Design review of the part built by this model. Coordinates are the model's own, in mm. Face numbers are marked on the shaded views. Give positions to 0.01 mm unless a question says otherwise; leave off trailing zeros. Loops run counter-clockwise (first coordinate to the right, second up) from the corner with the lowest first, then second, coordinate; pieces in that order, holes last. Notation, with made-up numbers: (-20, 88) -> (38, 88) arc R12 ccw to (38, 98) -> close; hole circle Ø11 at (18, 11). An arc over 180 degrees is marked (long way). Answer in a Markdown table with one row per item. Add a question column.
(1) Consider section D-D on x = -83. Write out the cut boundary in (y, z), then the cut area to 3 significant figures.
(2) Draft analysis for pull direction Y (two halves, no side actions). For the marked faces 1, 2 and 3, state which applies: +Y half, -Y half, draft (parallel to the pull), parting line (faces both ways), or undercut.
(3) Consider section B-B on x = -36.5. Write out the cut boundary in (y, z), then the cut area to 3 significant figures.
(4) Consider section A-A on y = -30. Write out the cut boundary in (x, z).
(5) For pin 1 (4 mm diameter, centred on x = 70.5, y = 35, fed in from -Z); pin 2 (4 mm diameter, centred on x = -32.5, y = 17.5, fed in from -Z); pin 3 (2 mm diameter, centred on y = -23.5, z = -3, fed in from +X), all flat-tipped, find the tip position at first contact; note any pin that passes through.
(6) For line 1 (Y direction, x = 32.5, z = 8.5); line 2 (Z direction, x = -15, y = 40.5); line 3 (X direction, y = 10.5, z = 6), list the stretches that pass through material, from the lowest coordinate up.
(7) Consider section C-C on y = 17. Write out the cut boundary in (x, z).
from build123d import *

# Parameters (mm, degrees)
BOSS_EXTRUDE1_DEPTH    = 13
SKETCH3_R              = 1.65
SKETCH3_R_2            = 1.5
CUT_EXTRUDE1_DEPTH     = 14
SKETCH4_W              = 13
SKETCH4_H              = 83
BOSS_EXTRUDE2_DEPTH    = 5
BOSS_EXTRUDE3_DEPTH    = 1
FILLET1_R              = 2
HOLE_WIZARD_M3_1_D     = 2.5
HOLE_WIZARD_M3_1_DEPTH = 12
HOLE_WIZARD_M3_1_TIP   = 0.751075774
CUT_EXTRUDE_1_DEPTH    = 17


with BuildPart() as part:
    # Sketch1 → Boss-Extrude1 (new body)
    with BuildSketch(Plane.XY):
        Polygon((-95, 44), (-35, 44), (95, 44), (95, -44), (-95, -44), align=None)
    extrude(amount=BOSS_EXTRUDE1_DEPTH)

    # Sketch3 → Cut-Extrude1 (cut, through all)
    with BuildSketch(Plane.XY.offset(13)):
        with Locations((-58.6, -41.5)):
            Circle(SKETCH3_R)
        with Locations((-23.6, -41.5)):
            Circle(SKETCH3_R)
        with Locations((11.4, -41.5)):
            Circle(SKETCH3_R)
        with Locations((32.5, -41.5)):
            Circle(SKETCH3_R_2)
        with Locations((77.5, -41.5)):
            Circle(SKETCH3_R_2)
    extrude(amount=-CUT_EXTRUDE1_DEPTH, mode=Mode.SUBTRACT)

    # Sketch4 → Boss-Extrude2 (add)
    with BuildSketch(Plane(origin=(0, 0, 0), x_dir=(-1, 0, 0), z_dir=(0, 0, -1))):
        with Locations((72, 2.5)):
            Rectangle(SKETCH4_W, SKETCH4_H)
    extrude(amount=BOSS_EXTRUDE2_DEPTH)

    # Sketch5 → Boss-Extrude3 (add)
    with BuildSketch(Plane(origin=(0, 0, 0), x_dir=(-1, 0, 0), z_dir=(0, 0, -1))):
        Polygon((65.5, -39), (-15, -39), (-15, -34), (-14, -34), (-14, -38), (65.5, -38), align=None)
    extrude(amount=BOSS_EXTRUDE3_DEPTH)

    # Fillet1
    fillet1_edges = [part.edges().sort_by_distance(p)[0] for p in [
        (14, -38, -0.5),
    ]]
    fillet(fillet1_edges, radius=FILLET1_R)

    # M3 螺纹孔1
    with Locations(Plane(origin=(-70.5, 44, 2.5), x_dir=(1, 0, 0), z_dir=(0, 1, 0))):
        with Locations((0, 0), (31, 0), (55.5, 0), (105.5, 0), (155.5, 0)):
            Hole(HOLE_WIZARD_M3_1_D / 2, depth=HOLE_WIZARD_M3_1_DEPTH)
            with Locations((0, 0, -(HOLE_WIZARD_M3_1_DEPTH + HOLE_WIZARD_M3_1_TIP / 2))):  # 118° drill point
                Cone(0, HOLE_WIZARD_M3_1_D / 2, HOLE_WIZARD_M3_1_TIP, mode=Mode.SUBTRACT)

    # 草图4 → 切除-拉伸1 (cut)
    with BuildSketch(Plane(origin=(0, 0, -5), x_dir=(-1, 0, 0), z_dir=(0, 0, -1))):
        with BuildLine():
            Line((29.5, 29), (29.5, 4))
            ThreePointArc((29.5, 4), (36.5, -3), (43.5, 4))
            Line((43.5, 4), (43.5, 29))
            ThreePointArc((43.5, 29), (36.5, 36), (29.5, 29))
        make_face()
    extrude(amount=-CUT_EXTRUDE_1_DEPTH, mode=Mode.SUBTRACT)


solid = part.part
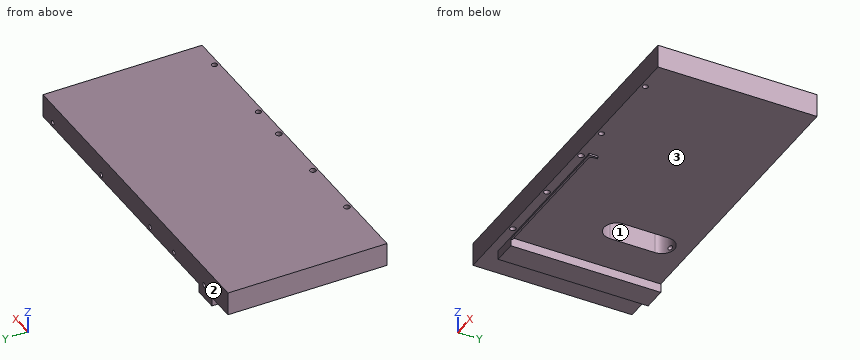
Values follow:
| question | item | result |
|---|---|---|
| 1 | outline | (-44, 0) -> (44, 0) -> (44, 13) -> (-44, 13) -> close |
| 1 | area | 1,140 mm2 |
| 2 | face 1 | undercut |
| 2 | face 2 | +Y half |
| 2 | face 3 | draft |
| 3 | outline | (-44, 0) -> (-39, 0) -> (-39, -1) -> (-38, -1) -> (-38, 0) -> (-3, 0) -> (-3, 12) -> (36, 12) -> (36, 0) -> (44, 0) -> (44, 13) -> (-44, 13) -> close |
| 3 | area | 677 mm2 |
| 4 | outline | (-95, 0) -> (-78.5, 0) -> (-78.5, -5) -> (-65.5, -5) -> (-65.5, 0) -> (95, 0) -> (95, 13) -> (-95, 13) -> close |
| 5 | pin 1 | z = 0 |
| 5 | pin 2 | z = 12 |
| 5 | pin 3 | x = -65.5 |
| 6 | line 1 | -44 to -43, -40 to 44 |
| 6 | line 2 | 0 to 1.25, 3.75 to 13 |
| 6 | line 3 | -95 to -43.5, -29.5 to 95 |
| 7 | outline | (-95, 0) -> (-78.5, 0) -> (-78.5, -5) -> (-65.5, -5) -> (-65.5, 0) -> (-43.5, 0) -> (-43.5, 12) -> (-29.5, 12) -> (-29.5, 0) -> (95, 0) -> (95, 13) -> (-95, 13) -> close |
